Here's how the part is built. I have some questions about the finished solid (model axes, mm). Face numbers are marked on the shaded views. Round coordinates to 2 decimals unless told otherwise and drop trailing zeros. Write each loop counter-clockwise with the first axis right and the second up, starting at its lowest first coordinate (ties: lowest second). Pieces come first, ordered by that corner, then holes. Notation, with made-up numbers: M -5.75,61 L 40.25,61 A29 ccw 40.25,86 Z; hole C -35,68.5 d2. An arc over 180 degrees is marked long. Use one line per item in the form item = value. Start each with the question number.
Q1. I want a section at D-D on x = 14.5. State how many separate pieces and enclosed holes the cut face has, and give its area (3 significant figures).
Q2. I want a section at A-A on y = 0. List the corners of the cut face in (x, z) for me.
Q3. I'm going to push flat-ended pins straight in: pin 1 Ø2.5 at (x, z) = (-28.5, 20.5) entering from -Y; pin 2 Ø1.5 at (x, z) = (14.5, 20.5) entering from +Y; pin 3 Ø1.5 at (x, z) = (-17, 16.5) entering from +Y. Where does each tip first touch, or does it pass through?
Q4. We'd pull the mould along Y, two halves only. Please class the marked faces 1, 2 and 3: +Y half, -Y half, draft (parallel to the pull), parting line (faces both ways), or undercut.
Q5. I want a section at B-B on z = 16.5. List the corners of the cut face in (x, y) for me, and give its area (3 significant figures).
Q6. I need wall thicknesses on line 1 along X through (y, z) = (0, 18.25); line 2 along Y through (x, z) = (30.5, 21). Which ranges of each line are inside material? Lowest first, please. Write a range as from..to.
```python
from build123d import *

# Parameters (mm, degrees)
CYLINDER063_R         = 50
CYLINDER063_DEPTH     = 10
CYLINDER067_R         = 37.5
CYLINDER067_DEPTH     = 5
CYLINDER059_R         = 45
CYLINDER059_DEPTH     = 5
BOX024_W              = 66
BOX024_H              = 4
BOX024_DEPTH          = 5
BOX028_W              = 66
BOX028_H              = 4
BOX028_DEPTH          = 5
BOX022_W              = 74
BOX022_H              = 4
BOX022_DEPTH          = 5
BOX020_W              = 74
BOX020_H              = 4
BOX020_DEPTH          = 5
BOX025_W              = 74
BOX025_H              = 4
BOX025_DEPTH          = 5
BOX027_W              = 66
BOX027_H              = 4
BOX027_DEPTH          = 5
BOX026_W              = 76
BOX026_H              = 4
BOX026_DEPTH          = 5
BOX021_W              = 66
BOX021_H              = 4
BOX021_DEPTH          = 5
BOX029_W              = 76
BOX029_H              = 4
BOX029_DEPTH          = 5
BOX023_W              = 74
BOX023_H              = 4
BOX023_DEPTH          = 5
CYLINDER065_R         = 37.3
CYLINDER065_DEPTH     = 5
CYLINDER060_R         = 37.5
CYLINDER060_DEPTH     = 5
SKETCH005_R           = 1.8
PAD001_DEPTH          = 0.6
POLARPATTERN003_COUNT = 4


with BuildPart() as cylinder063:
    # Cylinder063 → Cylinder063 (new body)
    with BuildSketch(Plane.XY.offset(-49)):
        Circle(CYLINDER063_R)
    extrude(amount=CYLINDER063_DEPTH)


with BuildPart() as cylinder067:
    # Cylinder067 → Cylinder067 (new body)
    with BuildSketch(Plane.XY.offset(-41)):
        Circle(CYLINDER067_R)
    extrude(amount=CYLINDER067_DEPTH)


with BuildPart() as cut032:
    # Cylinder059 → Cylinder059 (new body)
    with BuildSketch(Plane.XY.offset(-41)):
        Circle(CYLINDER059_R)
    extrude(amount=CYLINDER059_DEPTH)

    # Cut032: cut Cylinder067
    add(cylinder067.part, mode=Mode.SUBTRACT)


with BuildPart() as cube024:
    # Box024 → Box024 (new body)
    with BuildSketch(Plane(origin=(-18, -33, -41), x_dir=(0, 1, 0), z_dir=(0, 0, 1))):
        with Locations((33, 2)):
            Rectangle(BOX024_W, BOX024_H)
    extrude(amount=BOX024_DEPTH)


with BuildPart() as cube028:
    # Box028 → Box028 (new body)
    with BuildSketch(Plane(origin=(22, -33, -41), x_dir=(0, 1, 0), z_dir=(0, 0, 1))):
        with Locations((33, 2)):
            Rectangle(BOX028_W, BOX028_H)
    extrude(amount=BOX028_DEPTH)


with BuildPart() as cube022:
    # Box022 → Box022 (new body)
    with BuildSketch(Plane(origin=(-8, -37, -41), x_dir=(0, 1, 0), z_dir=(0, 0, 1))):
        with Locations((37, 2)):
            Rectangle(BOX022_W, BOX022_H)
    extrude(amount=BOX022_DEPTH)


with BuildPart() as cube020:
    # Box020 → Box020 (new body)
    with BuildSketch(Plane(origin=(-37, 8, -41), x_dir=(1, 0, 0), z_dir=(0, 0, 1))):
        with Locations((37, 2)):
            Rectangle(BOX020_W, BOX020_H)
    extrude(amount=BOX020_DEPTH)


with BuildPart() as cube025:
    # Box025 → Box025 (new body)
    with BuildSketch(Plane(origin=(-37, -12, -41), x_dir=(1, 0, 0), z_dir=(0, 0, 1))):
        with Locations((37, 2)):
            Rectangle(BOX025_W, BOX025_H)
    extrude(amount=BOX025_DEPTH)


with BuildPart() as cube027:
    # Box027 → Box027 (new body)
    with BuildSketch(Plane(origin=(-33, -22, -41), x_dir=(1, 0, 0), z_dir=(0, 0, 1))):
        with Locations((33, 2)):
            Rectangle(BOX027_W, BOX027_H)
    extrude(amount=BOX027_DEPTH)


with BuildPart() as cube026:
    # Box026 → Box026 (new body)
    with BuildSketch(Plane(origin=(-38, -2, -41), x_dir=(1, 0, 0), z_dir=(0, 0, 1))):
        with Locations((38, 2)):
            Rectangle(BOX026_W, BOX026_H)
    extrude(amount=BOX026_DEPTH)


with BuildPart() as cube021:
    # Box021 → Box021 (new body)
    with BuildSketch(Plane(origin=(-33, 18, -41), x_dir=(1, 0, 0), z_dir=(0, 0, 1))):
        with Locations((33, 2)):
            Rectangle(BOX021_W, BOX021_H)
    extrude(amount=BOX021_DEPTH)


with BuildPart() as cube029:
    # Box029 → Box029 (new body)
    with BuildSketch(Plane(origin=(2, -38, -41), x_dir=(0, 1, 0), z_dir=(0, 0, 1))):
        with Locations((38, 2)):
            Rectangle(BOX029_W, BOX029_H)
    extrude(amount=BOX029_DEPTH)


with BuildPart() as cube023:
    # Box023 → Box023 (new body)
    with BuildSketch(Plane(origin=(12, -37, -41), x_dir=(0, 1, 0), z_dir=(0, 0, 1))):
        with Locations((37, 2)):
            Rectangle(BOX023_W, BOX023_H)
    extrude(amount=BOX023_DEPTH)


with BuildPart() as cylinder065:
    # Cylinder065 → Cylinder065 (new body)
    with BuildSketch(Plane.XY.offset(-41)):
        Circle(CYLINDER065_R)
    extrude(amount=CYLINDER065_DEPTH)


with BuildPart() as obj1:
    # Cylinder060 → Cylinder060 (new body)
    with BuildSketch(Plane.XY.offset(-41)):
        Circle(CYLINDER060_R)
    extrude(amount=CYLINDER060_DEPTH)

    # Cut035: cut Cylinder065
    add(cylinder065.part, mode=Mode.SUBTRACT)

    # Fusion022: union Cube024, Cube028, Cube022, Cube020, Cube025, Cube027, Cube026, Cube021, Cube029, Cube023
    add(cube024.part)
    add(cube028.part)
    add(cube022.part)
    add(cube020.part)
    add(cube025.part)
    add(cube027.part)
    add(cube026.part)
    add(cube021.part)
    add(cube029.part)
    add(cube023.part)

    # Cut036: cut Cut032
    add(cut032.part, mode=Mode.SUBTRACT)

    # Cut034: cut Cylinder063
    add(cylinder063.part, mode=Mode.SUBTRACT)


with BuildPart() as obj1_1:
    # Cut034 placement: moved
    add(obj1.part.moved(Location((0, 0, 57.4))))


with BuildPart() as obj2:
    # Sketch006 → Revolution002 (revolve)
    with BuildSketch(Plane.XZ):
        Polygon((-36.85, 13.55), (-38.7, 13.55), (-38.7, 18.442992), (-42.15, 21.4), (-36.85, 21.4), align=None)
    revolve(axis=Axis((0, 0, 0), (0, 0, 1)))

    # Sketch005 (on Face1 of Revolution002) → Pad001 (new body)
    with BuildSketch(Plane(origin=(0, 0, 13.55), x_dir=(1, 0, 0), z_dir=(0, 0, -1))):
        with Locations((-38.7, 0)):
            Circle(SKETCH005_R)
    pad001 = extrude(amount=-PAD001_DEPTH)

    # PolarPattern003: Pad001 ×4 about axis
    polarpattern003_axis = Axis((0, 0, 13.55), (0, 0, -1))
    for i in range(1, POLARPATTERN003_COUNT):
        add(pad001.rotate(polarpattern003_axis, i * 360 / POLARPATTERN003_COUNT))

    # Fusion036: union obj1
    add(obj1_1.part)


solid = obj2.part
```
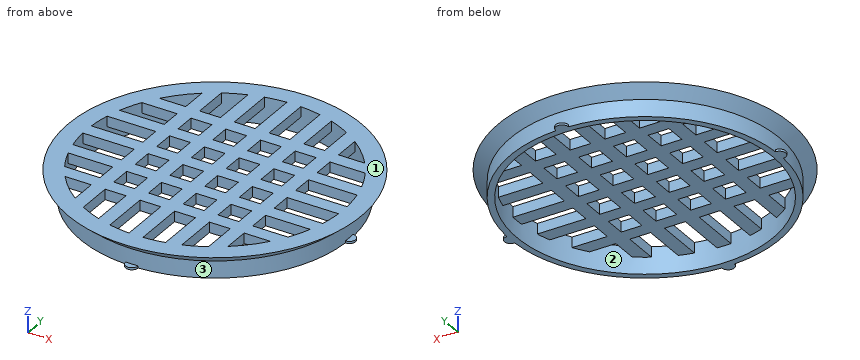
Reported:
q1.separate_pieces = 7
q1.enclosed_holes = 0
q1.area = 102 mm^2
q2.outline = M -42.15,21.4 L -38.7,18.44 L -38.7,14.15 L -40.5,14.15 L -40.5,13.55 L -36.85,13.55 L -36.85,18.4 L 36.85,18.4 L 36.85,13.55 L 40.5,13.55 L 40.5,14.15 L 38.7,14.15 L 38.7,18.44 L 42.15,21.4 Z
q3.pin_1 = -31.83
q3.pin_2 = 39.43
q3.pin_3 = 35.12
q4.face_1 = draft
q4.face_2 = undercut
q4.face_3 = parting line
q5.outline = C 0,0 d77.4; hole C 0,0 d73.7
q5.area = 439 mm^2
q6.line_1 = -38.7..-36.85, 36.85..38.7
q6.line_2 = -28.41..-18, -12..-8, -2..2, 8..12, 18..28.41
